```python
from build123d import *

# Parameters (mm, degrees)
SKETCH1_R                 = 2.5
BOSS_EXTRUDE1_DEPTH       = 9.3
BOSS_EXTRUDE2_START       = -1
SKETCH3_W                 = 1.627840772
SKETCH3_H                 = 5.944538132
BOSS_EXTRUDE2_DEPTH       = 4
CIRPATTERN1_COUNT         = 9
BOSS_EXTRUDE3_DEPTH       = 1
M2X0_4_TAPPED_HOLE1_D     = 1.6
M2X0_4_TAPPED_HOLE1_DEPTH = 1
SKETCH7_R                 = 0.75
CUT_EXTRUDE1_DEPTH        = 10.3


with BuildPart() as part:
    # Sketch1 → Boss-Extrude1 (new body)
    with BuildSketch(Plane(origin=(0, 0, 0), x_dir=(1, 0, 0), z_dir=(0, 1, 0))):
        Circle(SKETCH1_R)
    extrude(amount=BOSS_EXTRUDE1_DEPTH)

    # Sketch3 → Boss-Extrude2 (add)
    with BuildSketch(Plane(origin=(0, 9.3, 0), x_dir=(1, 0, 0), z_dir=(0, 1, 0)).offset(BOSS_EXTRUDE2_START)):
        with Locations((0, -2.972269066)):
            Rectangle(SKETCH3_W, SKETCH3_H)
    boss_extrude2 = extrude(amount=-BOSS_EXTRUDE2_DEPTH)

    # CirPattern1: Boss-Extrude2 ×9 about axis
    cirpattern1_axis = Axis((0, 0, 0), (0, 1, 0))
    for i in range(1, CIRPATTERN1_COUNT):
        add(boss_extrude2.rotate(cirpattern1_axis, i * 360 / CIRPATTERN1_COUNT))

    # Sketch4 → Boss-Extrude3 (add)
    with BuildSketch(Plane.XZ):
        with BuildLine():
            ThreePointArc((-1.942516625, 4.026805507), (-4.242640687, 4.242640687), (-4.026805507, 1.942516625))
            ThreePointArc((-4.026805507, 1.942516625), (-3, 0), (-4.026805507, -1.942516625))
            ThreePointArc((-4.026805507, -1.942516625), (-4.242640687, -4.242640687), (-1.942516625, -4.026805507))
            ThreePointArc((-1.942516625, -4.026805507), (0, -3), (1.942516625, -4.026805507))
            ThreePointArc((1.942516625, -4.026805507), (4.242640687, -4.242640687), (4.026805507, -1.942516625))
            ThreePointArc((4.026805507, -1.942516625), (3, 0), (4.026805507, 1.942516625))
            ThreePointArc((4.026805507, 1.942516625), (4.242640687, 4.242640687), (1.942516625, 4.026805507))
            ThreePointArc((1.942516625, 4.026805507), (0, 3), (-1.942516625, 4.026805507))
        make_face()
    extrude(amount=-BOSS_EXTRUDE3_DEPTH)

    # M2x0.4 Tapped Hole1
    with Locations(Plane(origin=(0, 0, 0), x_dir=(-1, 0, 0), z_dir=(0, -1, 0))):
        with Locations((3.181980515, 3.181980515), (-3.181980515, 3.181980515), (-3.181980515, -3.181980515), (3.181980515, -3.181980515)):
            Hole(M2X0_4_TAPPED_HOLE1_D / 2, depth=M2X0_4_TAPPED_HOLE1_DEPTH)

    # Sketch7 → Cut-Extrude1 (cut, through all)
    with BuildSketch(Plane.XZ):
        Circle(SKETCH7_R)
    extrude(amount=-CUT_EXTRUDE1_DEPTH, mode=Mode.SUBTRACT)


solid = part.part
```
Work out the finished part from the listing and answer in its coordinate system (mm). A direction names the side the tool comes from. Coordinates: 2 decimals unless noted, no trailing zeros. Write each loop counter-clockwise with the first axis right and the second up, starting at its lowest first coordinate (ties: lowest second). Pieces come first, ordered by that corner, then holes. Notation, with made-up numbers: (-11, 81) - (43, 81) arc R17 cw to (43, 87) - close; hole circle Ø11 at (-17, -19). An arc over 180 degrees is marked (long way). Answer as a JSON object with one key per item and string values.
Q1. For a pull along X with two mould halves and no side action, classify faces 5 (the flat face through (-5.142, 6.328, -2.982)), 6 (the flat face through (-3.212, 6.328, -2.794)), 7 (the flat face through (-0.665, 6.328, -4.206)), 8 (the flat face through (4, 4.3, -2)) as pulls with the +X half, pulls with the -X half, needs draft (parallel to the pull), parting line crosses it, or undercut.
Results list:
{"face 5": "pulls with the -X half", "face 6": "undercut", "face 7": "undercut", "face 8": "needs draft"}
Q2. Find section D-D (y = 1.75). Write down the section's boundary in (x, z), plus the area to 3 significant figures.
Results list:
{"outline": "circle Ø5 at (0, 0); hole circle Ø1.5 at (0, 0)", "area": "17.9 mm^2"}
Q3. Find section C-C (z = -2.75). Write down the section's boundary in (x, y).
Results list:
{"outline": "(-5.28, 4.3) - (-3.14, 4.3) - (-3.14, 8.3) - (-5.28, 8.3) - close; (-4.62, 0) - (-3.86, 0) - (-3.86, 1) - (-4.62, 1) - close; (-2.51, 0) - (2.51, 0) - (2.51, 1) - (-2.51, 1) - close; (-1.87, 4.3) - (-0.13, 4.3) - (-0.13, 8.3) - (-1.87, 8.3) - close; (0.13, 4.3) - (1.87, 4.3) - (1.87, 8.3) - (0.13, 8.3) - close; (3.14, 4.3) - (5.28, 4.3) - (5.28, 8.3) - (3.14, 8.3) - close; (3.86, 0) - (4.62, 0) - (4.62, 1) - (3.86, 1) - close"}
Q4. Consider L1, parallel to Y at x = 1.5, z = -2.25; L2, parallel to Z at x = 0, y = 3.25; L3, parallel to Y at x = -5, z = -2.75. Determine where each line is inside the solid, lowest interval first. Write a range as from..to.
Results list:
{"L1": "y = 0..1, 4.3..8.3", "L2": "z = -2.5..-0.75, 0.75..2.5", "L3": "y = 4.3..8.3"}
Q5. Which of the six approach directions +Z, -Z, +X, -X, +Y, -Y give full straight-line access (tool end or side, diameter ignored) to faces 1 (the flat face through (3, 4.3, 3)), 2 (the cylindrical face through (0, 0.5, -3)), 3 (the cylindrical face through (2.55, 0.51, 3.67)), 4 (the flat face through (-3, 8.3, 3))?
Results list:
{"face 1": "+Z, +X", "face 2": "-Z, -Y", "face 3": "-Y", "face 4": "+Z, -X, +Y"}
Q6. Find section A-A (z = 0). Write down the section's boundary in (x, y).
Results list:
{"outline": "(-4.69, 4.3) - (-2.5, 4.3) - (-2.5, 1) - (-3, 1) - (-3, 0) - (-0.75, 0) - (-0.75, 9.3) - (-2.5, 9.3) - (-2.5, 8.3) - (-4.69, 8.3) - close; (0.75, 0) - (3, 0) - (3, 1) - (2.5, 1) - (2.5, 4.3) - (4.69, 4.3) - (4.69, 8.3) - (2.5, 8.3) - (2.5, 9.3) - (0.75, 9.3) - close"}
Q7. Given pin 1 Ø0.7 at (x, z) = (-4.5, 1) entering from -Y; pin 2 Ø1.1 at (y, z) = (5.5, 5) entering from +X; pin 3 Ø2 at (y, z) = (5, 3.5) entering from -X, each flat-ended and moving along its own axis, determine where each tip first touches the part or whether it passes through.
Results list:
{"pin 1": "stops at y = 4.3", "pin 2": "stops at x = 3.94", "pin 3": "stops at x = -4.44"}
Q8. Find section B-B (x = -5). Write down the section's boundary in (y, z).
Results list:
{"outline": "(4.3, -3.23) - (8.3, -3.23) - (8.3, -1.95) - (4.3, -1.95) - close; (4.3, 0.06) - (8.3, 0.06) - (8.3, 1.71) - (4.3, 1.71) - close"}
